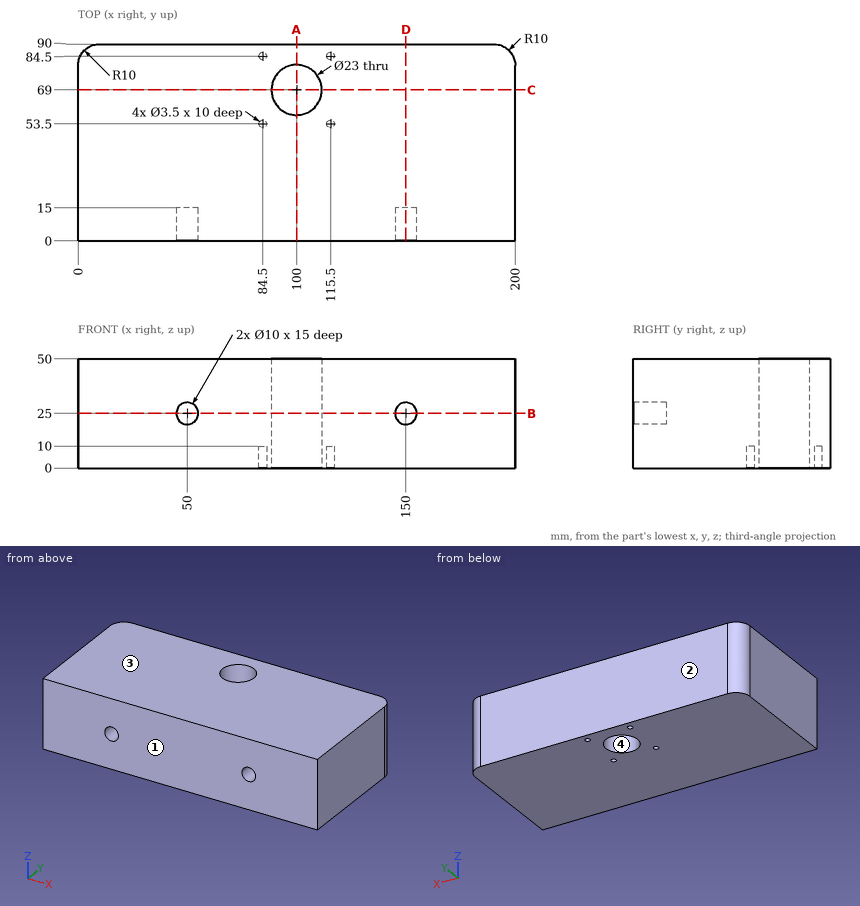
Could you check a few things on this drawing? It's one solid part, dimensions in mm from its lowest x, y, z. Give positions to 0.01 mm unless a question says otherwise; leave off trailing zeros. Order: outer loops, then holes, each group sorted by start corner. A loop starts at its lowest first (then second) coordinate and runs counter-clockwise, first axis right, second up. Notation, with made-up numbers: M -11,69.5 L 37,69.5 A9 ccw 37,78.5 Z; hole C 57.25,52 d7. An arc over 180 degrees is marked long. Use one line per item in the form item = value. Start each with the question number.
Item 1: If we section it at A-A (x = 100): Write out the boundary of the cut face in (y, z), then the cut area to 3 significant figures.
Item 2: We'd pull the mould along Y, two halves only. Please class the marked faces 1, 2, 3 and 4: +Y half, -Y half, draft (parallel to the pull), parting line (faces both ways), or undercut.
Item 3: If we section it at C-C (y = 69): Write out the boundary of the cut face in (x, z).
Item 4: If we section it at B-B (z = 25): Write out the boundary of the cut face in (x, y).
Item 5: If I drill on line 1 along Y through (x, z) = (115.5, 4); line 2 along Z through (x, y) = (50, 11.5); line 3 along X through (y, z) = (84, 7), over which ranges is the centre line in solid material (lowest first)?
Item 6: Will this pin go through, and if not, where does the flat tip stop? pin 1 Ø3 at (x, y) = (84.5, 84.5) entering from -Z.
Item 7: If we section it at D-D (x = 150): Write out the boundary of the cut face in (y, z).
Outcome:
q1.outline = M 0,0 L 57.5,0 L 57.5,50 L 0,50 Z; M 80.5,0 L 90,0 L 90,50 L 80.5,50 Z
q1.area = 3,350 mm2
q2.face_1 = -Y half
q2.face_2 = +Y half
q2.face_3 = draft
q2.face_4 = undercut
q3.outline = M 0,0 L 88.5,0 L 88.5,50 L 0,50 Z; M 111.5,0 L 200,0 L 200,50 L 111.5,50 Z
q4.outline = M 0,0 L 45,0 L 45,15 L 55,15 L 55,0 L 145,0 L 145,15 L 155,15 L 155,0 L 200,0 L 200,80 A10 ccw 190,90 L 10,90 A10 ccw 0,80 Z; hole C 100,69 d23
q5.line_1 = 0 to 51.75, 55.25 to 82.75, 86.25 to 90
q5.line_2 = 0 to 20, 30 to 50
q5.line_3 = 0.83 to 82.82, 86.18 to 113.82, 117.18 to 199.17
q6.pin_1 = 10
q7.outline = M 0,0 L 90,0 L 90,50 L 0,50 L 0,30 L 15,30 L 15,20 L 0,20 Z
